Design review of the part built by this model. Coordinates are the model's own, in mm. Face numbers are marked on the shaded views. A direction names the side the tool comes from. Coordinates: 2 decimals unless noted, no trailing zeros. Write each loop counter-clockwise with the first axis right and the second up, starting at its lowest first coordinate (ties: lowest second). Pieces come first, ordered by that corner, then holes. Notation, with made-up numbers: (-28.5, 35.25) -> (14.5, 35.25) arc R23 ccw to (14.5, 61.25) -> close; hole circle Ø9 at (81, -24.75). An arc over 180 degrees is marked (long way). Answer in a Markdown table with one row per item. Add a question column.
Item 1: For the marked faces 5 and 6, list the 3-axis set-ups (+Z, -Z, +X, -X, +Y, -Y) from which the entire face can be reached by the end or side of a thin tool; tool diameter is ignored.
Item 2: Take a section at B-B, the plane x = -184.5. Write out the cut boundary in (y, z) (3 decimals).
Item 3: Take a section at A-A, the plane y = 15.5. Write out the cut boundary in (x, z) (3 decimals).
Item 4: Clearance check with flat-ended pins moving along their axes: P1, Ø8.5, axis at x = 282.575, z = 95.25, coming from the +Y side; P2, Ø4, axis at y = 65.5, z = 57, coming from the +X side; P3, Ø8, axis at y = 42, z = 59.5, coming from the -X side. State where each tip first meets the part, or that it passes through.
Item 5: Draft analysis for pull direction Z (two halves, no side actions). For the marked faces 1, 2, 3 and 4, state which applies: released by +Z, released by -Z, zero draft, split by the parting line, or undercut.
Item 6: Take a section at C-C, the plane y = 45. Write out the cut boundary in (x, z) (3 decimals), and give its area (3 significant figures).
Item 7: Take a section at D-D, the plane x = 94. Write out the cut boundary in (y, z) (3 decimals).
Item 8: To check wall thickness, follow line 1 (Z direction, x = 211.5, y = 23.5) (3 decimals); line 2 (X direction, y = 11, z = 12); line 3 (Y direction, x = 244, z = 7.5) (3 decimals). State the ranges of each line that lie inside material, in increasing order.
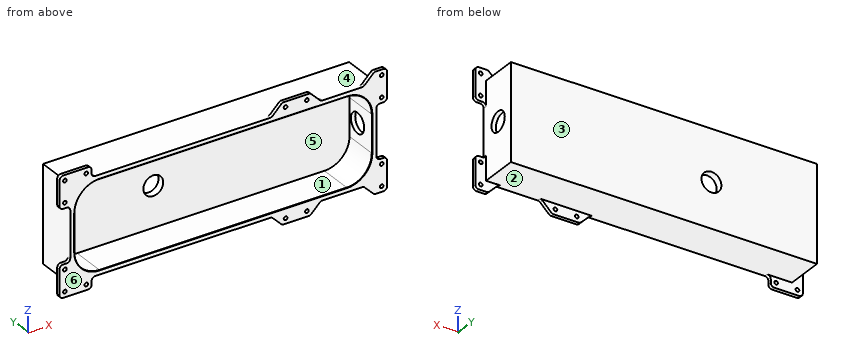
from build123d import *

# Parameters (mm, degrees)
SKETCH1_W           = 546.1
SKETCH1_H           = 171.45
BOSS_EXTRUDE1_DEPTH = 73.025
CUT_EXTRUDE1_DEPTH  = 60.325
CUT_EXTRUDE2_REACH  = 75.025
SKETCH5_R           = 17.749738032
CUT_EXTRUDE3_REACH  = 548.1
SKETCH6_R           = 17.749738032
CHAMFER1_SIZE       = 0.635
SKETCH7_R           = 3.2639
BOSS_EXTRUDE4_DEPTH = 6.35


with BuildPart() as part:
    # Sketch1 → Boss-Extrude1 (new body)
    with BuildSketch(Plane(origin=(0, 0, 0), x_dir=(1, 0, 0), z_dir=(0, 1, 0))):
        Rectangle(SKETCH1_W, SKETCH1_H)
    extrude(amount=BOSS_EXTRUDE1_DEPTH)

    # Sketch2 → Cut-Extrude1 (cut)
    with BuildSketch(Plane.XZ):
        with BuildLine():
            Line((220.748619551, 78.012946552), (-220.748619551, 78.012946552))
            ThreePointArc((-220.748619551, 78.012946552), (-252.278035042, 64.953035042), (-265.337946552, 33.423619551))
            Line((-265.337946552, 33.423619551), (-265.337946552, -33.423619551))
            ThreePointArc((-265.337946552, -33.423619551), (-252.278035042, -64.953035042), (-220.748619551, -78.012946552))
            Line((-220.748619551, -78.012946552), (220.748619551, -78.012946552))
            ThreePointArc((220.748619551, -78.012946552), (252.278035042, -64.953035042), (265.337946552, -33.423619551))
            Line((265.337946552, -33.423619551), (265.337946552, 33.423619551))
            ThreePointArc((265.337946552, 33.423619551), (252.278035042, 64.953035042), (220.748619551, 78.012946552))
        make_face()
    extrude(amount=-CUT_EXTRUDE1_DEPTH, mode=Mode.SUBTRACT)

    # Sketch5 → Cut-Extrude2 (cut, up to next)
    with BuildSketch(Plane(origin=(0, 73.025, 0), x_dir=(1, 0, 0), z_dir=(0, 1, 0)), mode=Mode.PRIVATE) as cut_extrude2_sk1:
        with Locations((-84.700666343, 5.811180929)):
            Circle(SKETCH5_R)
    cut_extrude2_tool1 = extrude(cut_extrude2_sk1.sketch, amount=-CUT_EXTRUDE2_REACH, mode=Mode.PRIVATE) & part.part
    add(cut_extrude2_tool1.solids().sort_by_distance((-84.700666, 73.025, -5.811181))[0], mode=Mode.SUBTRACT)

    # Sketch6 → Cut-Extrude3 (cut, up to next)
    with BuildSketch(Plane(origin=(273.05, 0, 0), x_dir=(0, 0, -1), z_dir=(1, 0, 0)), mode=Mode.PRIVATE) as cut_extrude3_sk1:
        with Locations((-0.077641224, 38.739963406)):
            Circle(SKETCH6_R)
    cut_extrude3_tool1 = extrude(cut_extrude3_sk1.sketch, amount=-CUT_EXTRUDE3_REACH, mode=Mode.PRIVATE) & part.part
    add(cut_extrude3_tool1.solids().sort_by_distance((273.05, 38.739963, 0.077641))[0], mode=Mode.SUBTRACT)

    # Chamfer1
    chamfer1_edges = [part.edges().sort_by_distance(p)[0] for p in [
        (252.278035042, 0, 64.953035042),
        (252.278035042, 0, -64.953035042),
        (-252.278035042, 0, -64.953035042),
        (0, 0, 78.012946552),
        (-252.278035042, 0, 64.953035042),
        (-265.337946552, 0, 0),
        (0, 0, -78.012946552),
        (265.337946552, 0, 0),
    ]]
    chamfer(chamfer1_edges, length=CHAMFER1_SIZE)

    # Sketch7 → Boss-Extrude4 (add)
    with BuildSketch(Plane.XZ):
        with BuildLine():
            ThreePointArc((-279.4, 47.625), (-274.909871939, 45.765128061), (-273.05, 41.275))
            Line((-273.05, 41.275), (-273.05, 85.725))
            Line((-273.05, 85.725), (-228.6, 85.725))
            ThreePointArc((-228.6, 85.725), (-233.090128061, 87.584871939), (-234.95, 92.075))
            Line((-234.95, 92.075), (-234.95, 98.425))
            ThreePointArc((-234.95, 98.425), (-236.809871939, 102.915128061), (-241.3, 104.775))
            Line((-241.3, 104.775), (-285.75, 104.775))
            ThreePointArc((-285.75, 104.775), (-290.240128061, 102.915128061), (-292.1, 98.425))
            Line((-292.1, 98.425), (-292.1, 53.975))
            ThreePointArc((-292.1, 53.975), (-290.240128061, 49.484871939), (-285.75, 47.625))
            Line((-285.75, 47.625), (-279.4, 47.625))
        make_face()
        with Locations((-282.575, 57.15)):
            Circle(SKETCH7_R, mode=Mode.SUBTRACT)
        with Locations((-282.575, 95.25)):
            Circle(SKETCH7_R, mode=Mode.SUBTRACT)
        with Locations((-244.475, 95.25)):
            Circle(SKETCH7_R, mode=Mode.SUBTRACT)
        with BuildLine():
            ThreePointArc((88.129615818, 87.584871939), (86.069527553, 86.208364969), (83.639487758, 85.725))
            Line((83.639487758, 85.725), (176.710512242, 85.725))
            ThreePointArc((176.710512242, 85.725), (174.280472447, 86.208364969), (172.220384182, 87.584871939))
            Line((172.220384182, 87.584871939), (156.890128061, 102.915128061))
            ThreePointArc((156.890128061, 102.915128061), (154.830039796, 104.291635031), (152.4, 104.775))
            Line((152.4, 104.775), (107.95, 104.775))
            ThreePointArc((107.95, 104.775), (105.519960204, 104.291635031), (103.459871939, 102.915128061))
            Line((103.459871939, 102.915128061), (88.129615818, 87.584871939))
        make_face()
        with Locations((111.125, 95.25)):
            Circle(SKETCH7_R, mode=Mode.SUBTRACT)
        with Locations((149.225, 95.25)):
            Circle(SKETCH7_R, mode=Mode.SUBTRACT)
        with BuildLine():
            ThreePointArc((252.140128061, 87.584871939), (250.080039796, 86.208364969), (247.65, 85.725))
            Line((247.65, 85.725), (273.05, 85.725))
            Line((273.05, 85.725), (273.05, 41.275))
            ThreePointArc((273.05, 41.275), (274.909871939, 45.765128061), (279.4, 47.625))
            Line((279.4, 47.625), (285.75, 47.625))
            ThreePointArc((285.75, 47.625), (290.240128061, 49.484871939), (292.1, 53.975))
            Line((292.1, 53.975), (292.1, 98.425))
            ThreePointArc((292.1, 98.425), (290.240128061, 102.915128061), (285.75, 104.775))
            Line((285.75, 104.775), (271.960512242, 104.775))
            ThreePointArc((271.960512242, 104.775), (269.530472447, 104.291635031), (267.470384182, 102.915128061))
            Line((267.470384182, 102.915128061), (252.140128061, 87.584871939))
        make_face()
        with Locations((282.575, 57.15)):
            Circle(SKETCH7_R, mode=Mode.SUBTRACT)
        with Locations((282.575, 95.25)):
            Circle(SKETCH7_R, mode=Mode.SUBTRACT)
        with BuildLine():
            Line((273.05, -85.725), (247.65, -85.725))
            ThreePointArc((247.65, -85.725), (250.080039796, -86.208364969), (252.140128061, -87.584871939))
            Line((252.140128061, -87.584871939), (267.470384182, -102.915128061))
            ThreePointArc((267.470384182, -102.915128061), (269.530472447, -104.291635031), (271.960512242, -104.775))
            Line((271.960512242, -104.775), (285.75, -104.775))
            ThreePointArc((285.75, -104.775), (290.240128061, -102.915128061), (292.1, -98.425))
            Line((292.1, -98.425), (292.1, -53.975))
            ThreePointArc((292.1, -53.975), (290.240128061, -49.484871939), (285.75, -47.625))
            Line((285.75, -47.625), (279.4, -47.625))
            ThreePointArc((279.4, -47.625), (274.909871939, -45.765128061), (273.05, -41.275))
            Line((273.05, -41.275), (273.05, -85.725))
        make_face()
        with Locations((282.575, -95.25)):
            Circle(SKETCH7_R, mode=Mode.SUBTRACT)
        with Locations((282.575, -57.15)):
            Circle(SKETCH7_R, mode=Mode.SUBTRACT)
        with BuildLine():
            Line((176.710512242, -85.725), (83.639487758, -85.725))
            ThreePointArc((83.639487758, -85.725), (86.069527553, -86.208364969), (88.129615818, -87.584871939))
            Line((88.129615818, -87.584871939), (103.459871939, -102.915128061))
            ThreePointArc((103.459871939, -102.915128061), (105.519960204, -104.291635031), (107.95, -104.775))
            Line((107.95, -104.775), (152.4, -104.775))
            ThreePointArc((152.4, -104.775), (154.830039796, -104.291635031), (156.890128061, -102.915128061))
            Line((156.890128061, -102.915128061), (172.220384182, -87.584871939))
            ThreePointArc((172.220384182, -87.584871939), (174.280472447, -86.208364969), (176.710512242, -85.725))
        make_face()
        with Locations((111.125, -95.25)):
            Circle(SKETCH7_R, mode=Mode.SUBTRACT)
        with Locations((149.225, -95.25)):
            Circle(SKETCH7_R, mode=Mode.SUBTRACT)
        with BuildLine():
            Line((-228.6, -85.725), (-273.05, -85.725))
            Line((-273.05, -85.725), (-273.05, -41.275))
            ThreePointArc((-273.05, -41.275), (-274.909871939, -45.765128061), (-279.4, -47.625))
            Line((-279.4, -47.625), (-285.75, -47.625))
            ThreePointArc((-285.75, -47.625), (-290.240128061, -49.484871939), (-292.1, -53.975))
            Line((-292.1, -53.975), (-292.1, -98.425))
            ThreePointArc((-292.1, -98.425), (-290.240128061, -102.915128061), (-285.75, -104.775))
            Line((-285.75, -104.775), (-241.3, -104.775))
            ThreePointArc((-241.3, -104.775), (-236.809871939, -102.915128061), (-234.95, -98.425))
            Line((-234.95, -98.425), (-234.95, -92.075))
            ThreePointArc((-234.95, -92.075), (-233.090128061, -87.584871939), (-228.6, -85.725))
        make_face()
        with Locations((-282.575, -95.25)):
            Circle(SKETCH7_R, mode=Mode.SUBTRACT)
        with Locations((-244.475, -95.25)):
            Circle(SKETCH7_R, mode=Mode.SUBTRACT)
        with Locations((-282.575, -57.15)):
            Circle(SKETCH7_R, mode=Mode.SUBTRACT)
    extrude(amount=-BOSS_EXTRUDE4_DEPTH)


solid = part.part
Answers:
| question | item | result |
|---|---|---|
| 1 | face 5 | -Y |
| 1 | face 6 | +Z, -Z, +X, -X, -Y |
| 2 | outline | (0, -85.725) -> (73.025, -85.725) -> (73.025, 85.725) -> (0, 85.725) -> (0, 78.648) -> (0.635, 78.013) -> (60.325, 78.013) -> (60.325, -78.013) -> (0.635, -78.013) -> (0, -78.648) -> close |
| 3 | outline | (-273.05, -85.725) -> (273.05, -85.725) -> (273.05, 85.725) -> (-273.05, 85.725) -> close; hole (-265.338, -33.424) arc R44.589 ccw to (-220.749, -78.013) -> (220.749, -78.013) arc R44.589 ccw to (265.338, -33.424) -> (265.338, 33.424) arc R44.589 ccw to (220.749, 78.013) -> (-220.749, 78.013) arc R44.589 ccw to (-265.338, 33.424) -> close |
| 4 | P1 | stops at y = 6.35 |
| 4 | P2 | stops at x = 273.05 |
| 4 | P3 | stops at x = -273.05 |
| 5 | face 1 | undercut |
| 5 | face 2 | released by -Z |
| 5 | face 3 | zero draft |
| 5 | face 4 | released by +Z |
| 6 | outline | (-273.05, -85.725) -> (273.05, -85.725) -> (273.05, -16.532) -> (265.338, -16.532) -> (265.338, -33.424) arc R44.589 cw to (220.749, -78.013) -> (-220.749, -78.013) arc R44.589 cw to (-265.338, -33.424) -> (-265.338, 33.424) arc R44.589 cw to (-220.749, 78.013) -> (220.749, 78.013) arc R44.589 cw to (265.338, 33.424) -> (265.338, 16.687) -> (273.05, 16.687) -> (273.05, 85.725) -> (-273.05, 85.725) -> close |
| 6 | area | 12,300 mm^2 |
| 7 | outline | (0, -93.455) -> (6.35, -93.455) -> (6.35, -85.725) -> (73.025, -85.725) -> (73.025, 85.725) -> (6.35, 85.725) -> (6.35, 93.455) -> (0, 93.455) -> (0, 78.648) -> (0.635, 78.013) -> (60.325, 78.013) -> (60.325, -78.013) -> (0.635, -78.013) -> (0, -78.648) -> close |
| 8 | line 1 | z = -85.725 to -78.013, 78.013 to 85.725 |
| 8 | line 2 | x = -273.05 to -265.34, 265.34 to 273.05 |
| 8 | line 3 | y = 60.325 to 73.025 |
